Input: part model. Units: mm. Frame: model coordinates. Give positions to 0.01 mm unless a question says otherwise; leave off trailing zeros. Write each loop counter-clockwise with the first axis right and the second up, starting at its lowest first coordinate (ties: lowest second). Pieces come first, ordered by that corner, then holes.
```python
from build123d import *

# Parameters (mm, degrees)
SKETCH1_R           = 0.5
BOSS_EXTRUDE1_DEPTH = 1.4
SKETCH2_R           = 2.35
CUT_EXTRUDE1_DEPTH  = 1
SKETCH3_R           = 3.5
SKETCH3_R_2         = 2.45
BOSS_EXTRUDE2_DEPTH = 2.5
SKETCH4_R           = 1.2
CUT_EXTRUDE2_DEPTH  = 20.282440198
SKETCH5_R           = 2.45
SKETCH5_R_2         = 1.2
BOSS_EXTRUDE3_DEPTH = 0.1
SKETCH6_W           = 35.735260114
SKETCH6_H           = 17.672039004
CUT_EXTRUDE4_DEPTH  = 20.513392837
CUT_EXTRUDE5_DEPTH  = 18.980545042
CIRPATTERN2_COUNT   = 2
SKETCH9_R           = 1.2
CUT_EXTRUDE6_DEPTH  = 20.282440198


with BuildPart() as part:
    # Sketch1 → Boss-Extrude1 (new body)
    with BuildSketch(Plane(origin=(0, 0, 0), x_dir=(1, 0, 0), z_dir=(0, 1, 0))):
        with BuildLine():
            Line((-15.2, 2), (-2, 2.95))
            Line((-2, 2.95), (-2, 6.35))
            ThreePointArc((-2, 6.35), (0, 8.35), (2, 6.35))
            Line((2, 6.35), (2, 3.5))
            Line((2, 3.5), (15.2, 2))
            ThreePointArc((15.2, 2), (17.2, 0), (15.2, -2))
            Line((15.2, -2), (2, -3.5))
            Line((2, -3.5), (2, -6.35))
            ThreePointArc((2, -6.35), (0, -8.35), (-2, -6.35))
            Line((-2, -6.35), (-2, -2.95))
            Line((-2, -2.95), (-15.2, -2))
            ThreePointArc((-15.2, -2), (-17.2, 0), (-15.2, 2))
        make_face()
        with Locations(Location((0, 6.35, 0), (0, 0, 270))):
            Circle(SKETCH1_R, mode=Mode.SUBTRACT)
        with Locations(Location((0, 4.55, 0), (0, 0, 270))):
            Circle(SKETCH1_R, mode=Mode.SUBTRACT)
        with Locations(Location((0, -4.55, 0), (0, 0, 90))):
            Circle(SKETCH1_R, mode=Mode.SUBTRACT)
        with Locations(Location((0, -6.35, 0), (0, 0, 90))):
            Circle(SKETCH1_R, mode=Mode.SUBTRACT)
        with Locations(Location((-15.2, 0, 0), (0, 0, 270))):
            Circle(SKETCH1_R, mode=Mode.SUBTRACT)
        with Locations(Location((15.2, 0, 0), (0, 0, 270))):
            Circle(SKETCH1_R, mode=Mode.SUBTRACT)
        with Locations(Location((-13.4, 0, 0), (0, 0, 270))):
            Circle(SKETCH1_R, mode=Mode.SUBTRACT)
        with Locations(Location((-11.6, 0, 0), (0, 0, 270))):
            Circle(SKETCH1_R, mode=Mode.SUBTRACT)
        with Locations(Location((-9.8, 0, 0), (0, 0, 270))):
            Circle(SKETCH1_R, mode=Mode.SUBTRACT)
        with Locations(Location((-8, 0, 0), (0, 0, 270))):
            Circle(SKETCH1_R, mode=Mode.SUBTRACT)
        with Locations(Location((-6.2, 0, 0), (0, 0, 270))):
            Circle(SKETCH1_R, mode=Mode.SUBTRACT)
        with Locations(Location((-4.4, 0, 0), (0, 0, 270))):
            Circle(SKETCH1_R, mode=Mode.SUBTRACT)
        with Locations(Location((13.4, 0, 0), (0, 0, 270))):
            Circle(SKETCH1_R, mode=Mode.SUBTRACT)
        with Locations(Location((11.6, 0, 0), (0, 0, 270))):
            Circle(SKETCH1_R, mode=Mode.SUBTRACT)
        with Locations(Location((9.8, 0, 0), (0, 0, 270))):
            Circle(SKETCH1_R, mode=Mode.SUBTRACT)
        with Locations(Location((8, 0, 0), (0, 0, 270))):
            Circle(SKETCH1_R, mode=Mode.SUBTRACT)
        with Locations(Location((6.2, 0, 0), (0, 0, 270))):
            Circle(SKETCH1_R, mode=Mode.SUBTRACT)
        with Locations(Location((4.4, 0, 0), (0, 0, 270))):
            Circle(SKETCH1_R, mode=Mode.SUBTRACT)
    boss_extrude1 = extrude(amount=BOSS_EXTRUDE1_DEPTH)

    # Sketch2 → Cut-Extrude1 (cut)
    with BuildSketch(Plane.XZ):
        with Locations(Location((0, 0, 0), (0, 0, 270))):
            Circle(SKETCH2_R)
    extrude(amount=-CUT_EXTRUDE1_DEPTH, mode=Mode.SUBTRACT)

    # Sketch3 → Boss-Extrude2 (add)
    with BuildSketch(Plane(origin=(0, 1.4, 0), x_dir=(1, 0, 0), z_dir=(0, 1, 0))):
        with Locations(Location((0, 0, 0), (0, 0, 270))):
            Circle(SKETCH3_R)
        with Locations(Location((0, 0, 0), (0, 0, 270))):
            Circle(SKETCH3_R_2, mode=Mode.SUBTRACT)
    extrude(amount=BOSS_EXTRUDE2_DEPTH)

    # Sketch4 → Cut-Extrude2 (cut, through all)
    with BuildSketch(Plane(origin=(0, 1.4, 0), x_dir=(1, 0, 0), z_dir=(0, 1, 0))):
        with Locations(Location((0, 0, 0), (0, 0, 270))):
            Circle(SKETCH4_R)
    extrude(amount=-CUT_EXTRUDE2_DEPTH, mode=Mode.SUBTRACT)

    # Sketch5 → Boss-Extrude3 (add)
    with BuildSketch(Plane(origin=(0, 1.4, 0), x_dir=(1, 0, 0), z_dir=(0, 1, 0))):
        with Locations(Location((0, 0, 0), (0, 0, 270))):
            Circle(SKETCH5_R)
        with Locations(Location((0, 0, 0), (0, 0, 270))):
            Circle(SKETCH5_R_2, mode=Mode.SUBTRACT)
    extrude(amount=BOSS_EXTRUDE3_DEPTH)

    # Sketch6 → Cut-Extrude4 (cut, through all)
    with BuildSketch(Plane.XZ):
        Rectangle(SKETCH6_W, SKETCH6_H)
        with BuildLine():
            Line((-1.868584713, -2.959457918), (-15.2, -2))
            ThreePointArc((-15.2, -2), (-17.2, 0), (-15.2, 2))
            Line((-15.2, 2), (-1.868584713, 2.959457918))
            ThreePointArc((-1.868584713, 2.959457918), (0, 3.5), (1.868584713, 2.959457918))
            Line((1.868584713, 2.959457918), (15.2, 2))
            ThreePointArc((15.2, 2), (17.2, 0), (15.2, -2))
            Line((15.2, -2), (1.868584713, -2.959457918))
            ThreePointArc((1.868584713, -2.959457918), (0, -3.5), (-1.868584713, -2.959457918))
        make_face(mode=Mode.SUBTRACT)
    extrude(amount=-CUT_EXTRUDE4_DEPTH, mode=Mode.SUBTRACT)

    # Sketch7 → Cut-Extrude5 (cut, through all)
    with BuildSketch(Plane.XZ):
        with BuildLine():
            Line((0, 3.5), (-17.731768104, 3.5))
            Line((-17.731768104, 3.5), (-17.731768104, -3.5))
            Line((-17.731768104, -3.5), (0, -3.5))
            ThreePointArc((0, -3.5), (-3.5, 0), (0, 3.5))
        make_face()
    extrude(amount=-CUT_EXTRUDE5_DEPTH, mode=Mode.SUBTRACT)

    # CirPattern2: Boss-Extrude1 ×2 about axis
    cirpattern2_axis = Axis((0, 0, 0), (0, 1, 0))
    for i in range(1, CIRPATTERN2_COUNT):
        add(boss_extrude1.rotate(cirpattern2_axis, i * 360 / CIRPATTERN2_COUNT))

    # Sketch9 → Cut-Extrude6 (cut, through all)
    with BuildSketch(Plane(origin=(0, 1.4, 0), x_dir=(1, 0, 0), z_dir=(0, 1, 0))):
        with Locations(Location((0, 0, 0), (0, 0, 270))):
            Circle(SKETCH9_R)
    extrude(amount=-CUT_EXTRUDE6_DEPTH, mode=Mode.SUBTRACT)


solid = part.part
```
Q1. Section C-C, the plane x = -4.4. Return the cut outline in (y, z).
Q2. Pin query (flat end, axial travel): pin 1 (4 mm diameter, centred on x = 0, z = 0, fed in from +Y); pin 2 (0.7 mm diameter, centred on y = 1, z = 4.5, fed in from -X); pin 3 (2 mm diameter, centred on x = 2.5, z = 4.5, fed in from +Y); pin 4 (1.9 mm diameter, centred on x = 0, z = 0, fed in from -Y). Return the tip coordinate at first contact, or that it passes through.
Q3. Material intervals for line 1 along Z through (x, y) = (15.2, 0.35); line 2 along Z through (x, y) = (-11.6, 0.65), sorted ascending.
Q4. Section A-A, the plane x = 8. Return the cut outline in (y, z).
Q5. Section B-B, the plane y = 2. Return the cut outline in (x, z).
Q6. Mould query, pull axis X, two halves, no side actions, for faces 1 (the flat face through (2, 1, -5)), 2 (the flat face through (-2, 1, -5)), 3 (the flat face through (-1, 1.5, -1)), 4 (the cylindrical face through (0.04, 0.69, 8.35)). Classes: +X half, -X half, draft (parallel to the pull), parting line (faces both ways), or undercut.
Solutions:
1. outline: (0, -3.23) - (1.4, -3.23) - (1.4, -0.5) - (0, -0.5) - close; (0, 0.5) - (1.4, 0.5) - (1.4, 3.23) - (0, 3.23) - close
2. pin 1: stops at y = 1.5
2. pin 2: stops at x = -2
2. pin 3: stops at y = 1.4
2. pin 4: passes through
3. line 1: z = -2 to -0.5, 0.5 to 2
3. line 2: z = -2.41 to -0.5, 0.5 to 2.41
4. outline: (0, -2.52) - (1.4, -2.52) - (1.4, -0.5) - (0, -0.5) - close; (0, 0.5) - (1.4, 0.5) - (1.4, 2.52) - (0, 2.52) - close
5. outline: circle Ø7 at (0, 0); hole circle Ø4.9 at (0, 0)
6. face 1: +X half
6. face 2: -X half
6. face 3: undercut
6. face 4: parting line
